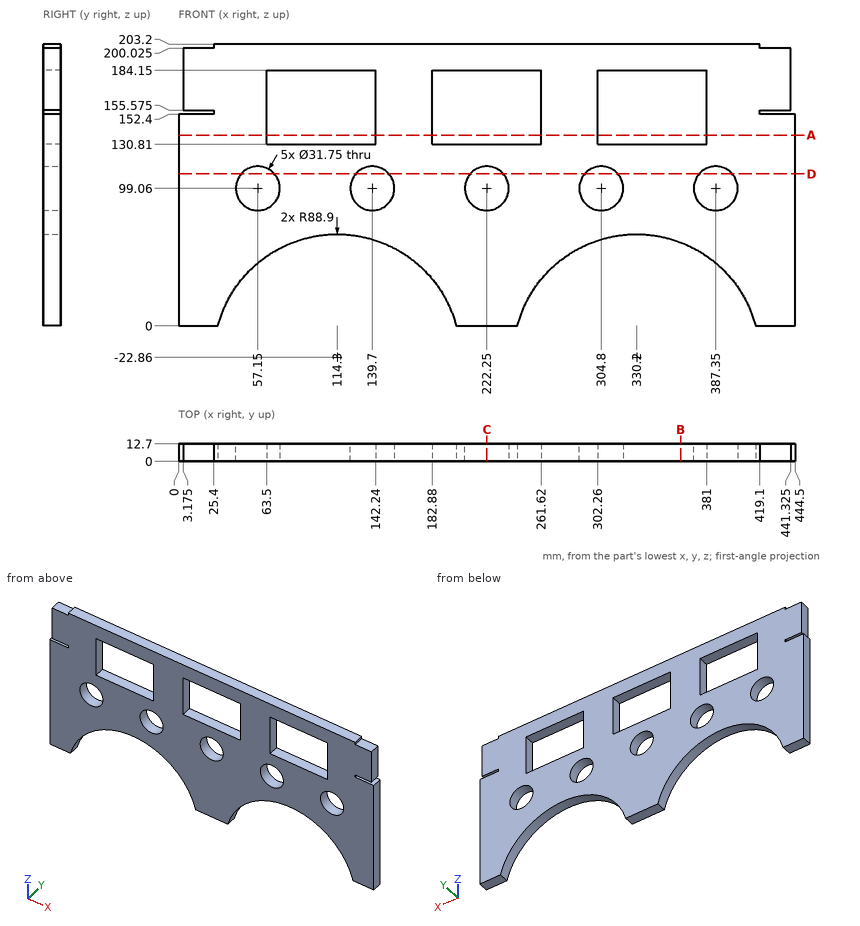
Job drawing, mm, ordinate dimensions from the low corner. One solid piece. Coordinates: 2 decimals unless noted, no trailing zeros. Order: outer loops, then holes, each group sorted by start corner. A loop starts at its lowest first (then second) coordinate and runs counter-clockwise, first axis right, second up. Notation, with made-up numbers: (13.25, 80.5) - (40.25, 80.5) arc R15 cw to (40.25, 92.5) - close; hole circle Ø4 at (-36, -26.75). An arc over 180 degrees is marked (long way). Write each question's results on one line, items separated by ' | '. Start each with the question number.
Item 1: Band-saw the part on B-B on x = 362. Write the cut outline in (y, z).
Item 2: Wall check: probe 1 along X at (y, z) = (6.5, 156) (3 decimals); probe 2 along Z at (x, y) = (222.25, 9.5) (3 decimals); probe 3 along Z at (x, y) = (139.7, 10.25) (3 decimals). Give the ranges that are in metal, low to high. Write a range as [from, to].
Item 3: Band-saw the part on A-A on z = 137.5. Write the cut outline in (x, y).
Item 4: Band-saw the part on D-D on z = 109.5. Write the cut outline in (x, y), and give its area (3 significant figures).
Item 5: Band-saw the part on C-C on x = 222.25. Write the cut outline in (y, z) (3 decimals), and give its area (3 significant figures).
Item 6: Flat gauge pins, fed straight in: pin 1 (4 mm diameter, centred on y = 11, z = 30, fed in from -X); pin 2 (6.5 mm diameter, centred on x = 435, y = 4, fed in from +Z) (3 decimals); pin 3 (3.5 mm diameter, centred on y = 7, z = 202, fed in from +X); pin 4 (2.5 mm diameter, centred on y = 9.5, z = 154.5, fed in from -X) (3 decimals). Where does each tip first touch, or does it go through?
Numbers:
1) outline: (0, 60.16) - (12.7, 60.16) - (12.7, 130.81) - (0, 130.81) - close; (0, 184.15) - (12.7, 184.15) - (12.7, 203.2) - (0, 203.2) - close
2) probe 1: [3.175, 63.5], [142.24, 182.88], [261.62, 302.26], [381, 441.325] | probe 2: [0, 83.185], [114.935, 130.81], [184.15, 203.2] | probe 3: [62.334, 83.185], [114.935, 130.81], [184.15, 203.2]
3) outline: (0, 0) - (63.5, 0) - (63.5, 12.7) - (0, 12.7) - close; (142.24, 0) - (182.88, 0) - (182.88, 12.7) - (142.24, 12.7) - close; (261.62, 0) - (302.26, 0) - (302.26, 12.7) - (261.62, 12.7) - close; (381, 0) - (444.5, 0) - (444.5, 12.7) - (381, 12.7) - close
4) outline: (0, 0) - (45.19, 0) - (45.19, 12.7) - (0, 12.7) - close; (69.11, 0) - (127.74, 0) - (127.74, 12.7) - (69.11, 12.7) - close; (151.66, 0) - (210.29, 0) - (210.29, 12.7) - (151.66, 12.7) - close; (234.21, 0) - (292.84, 0) - (292.84, 12.7) - (234.21, 12.7) - close; (316.76, 0) - (375.39, 0) - (375.39, 12.7) - (316.76, 12.7) - close; (399.31, 0) - (444.5, 0) - (444.5, 12.7) - (399.31, 12.7) - close | area: 4,130 mm^2
5) outline: (0, 0) - (12.7, 0) - (12.7, 83.185) - (0, 83.185) - close; (0, 114.935) - (12.7, 114.935) - (12.7, 130.81) - (0, 130.81) - close; (0, 184.15) - (12.7, 184.15) - (12.7, 203.2) - (0, 203.2) - close | area: 1,500 mm^2
6) pin 1: x = 0 | pin 2: z = 200.025 | pin 3: x = 419.1 | pin 4: x = 3.175
